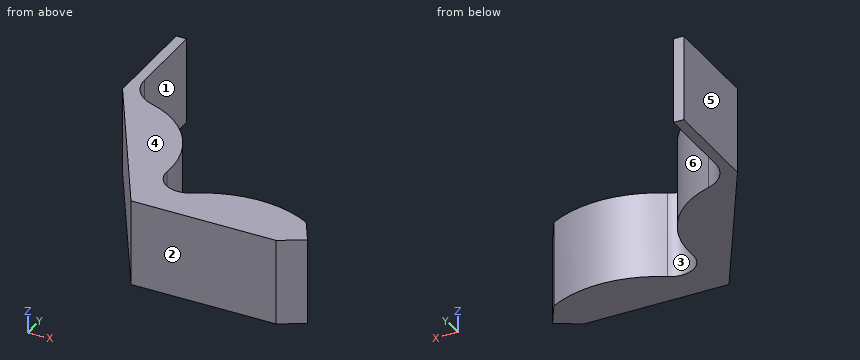
```python
from build123d import *

# Parameters (mm, degrees)
BOSS_EXTRUDE1_DEPTH = 250


with BuildPart() as part:
    # Sketch2 → Boss-Extrude1 (new body)
    with BuildSketch(Plane.XY):
        with BuildLine():
            Line((-277.128129211, 480), (0, 0))
            Line((0, 0), (420, 0))
            Line((420, 0), (489.282032303, 40))
            Line((489.282032303, 40), (445.980762114, 115))
            ThreePointArc((445.980762114, 115), (282.530694349, 155.502719239), (121.149011162, 107.415847331))
            ThreePointArc((121.149011162, 107.415847331), (48.13293846, 106.892445498), (14.374916134, 171.638231083))
            ThreePointArc((14.374916134, 171.638231083), (-32.686291511, 343.220804781), (-176.282688884, 448.270371763))
            ThreePointArc((-176.282688884, 448.270371763), (-227.488119154, 484.4090757), (-247.128129211, 543.926065009))
            Line((-247.128129211, 543.926065009), (-247.128129211, 775))
            Line((-247.128129211, 775), (-277.128129211, 775))
            Line((-277.128129211, 775), (-277.128129211, 480))
        make_face()
    extrude(amount=BOSS_EXTRUDE1_DEPTH)


solid = part.part
```
Source: CAD feature listing. Evaluate the final solid. Frame: model axes, mm. Face numbers are marked on the shaded views. A direction names the side the tool comes from. Coordinates: 2 decimals unless noted, no trailing zeros. Write each loop counter-clockwise with the first axis right and the second up, starting at its lowest first coordinate (ties: lowest second). Pieces come first, ordered by that corner, then holes. Notation, with made-up numbers: (-18.75, -38) -> (14.25, -38) arc R20 cw to (14.25, -13) -> close; hole circle Ø11 at (7, -12.75). An arc over 180 degrees is marked (long way). Return JSON: item names as keys, results as strings. Group by question number.
1) Section query A-A, the plane z = 121. Return loops of the section in (x, y), plus the area to 3 significant figures.
2) Ray query, line 1 along X through (y, z) = (583.5, 91); line 2 along Y through (x, z) = (89.5, 203.5); line 3 along X through (y, z) = (480, 120). Return the intervals inside material, ascending.
3) Section query B-B, the plane y = 564. Return loops of the section in (x, z).
4) Section query C-C, the plane x = 60. Return loops of the section in (y, z), plus the area to 3 significant figures.
5) Contact query for flat-ended pins moving along their axis: P1, Ø1.5, axis at x = 182.5, z = 128.5, coming from the +Y side; P2, Ø8, axis at y = 80.5, z = 190, coming from the +X side; P3, Ø2, axis at x = 203.5, z = 202.5, coming from the +Y side. Output: stop coordinate, or through.
6) Mould query, pull axis X, two halves, no side actions, for the marked faces 3, 4, 5 and 6. Classes: +X half, -X half, draft (parallel to the pull), parting line (faces both ways), or undercut.
7) Set-up query: the marked faces 1 and 2. Return all of +Z, -Z, +X, -X, +Y, -Y with unobstructed straight access to the full face (end or side cutting, diameter ignored); none if empty.
From the geometry:
{
 "1": {"outline": "(-277.13, 480) -> (0, 0) -> (420, 0) -> (489.28, 40) -> (445.98, 115) arc R320 ccw to (121.15, 107.42) arc R70 cw to (14.37, 171.64) arc R270 ccw to (-176.28, 448.27) arc R100 cw to (-247.13, 543.93) -> (-247.13, 775) -> (-277.13, 775) -> close", "area": "122,000 mm²"},
 "2": {"line 1": "-277.13 to -247.13", "line 2": "0 to 97.08", "line 3": "-277.13 to -224.03"},
 "3": {"outline": "(-277.13, 0) -> (-247.13, 0) -> (-247.13, 250) -> (-277.13, 250) -> close"},
 "4": {"outline": "(0, 0) -> (101.2, 0) -> (101.2, 250) -> (0, 250) -> close", "area": "25,300 mm²"},
 "5": {"P1": "y = 137.26", "P2": "x = 468.21", "P3": "y = 143.96"},
 "6": {"face 3": "undercut", "face 4": "draft", "face 5": "-X half", "face 6": "+X half"},
 "7": {"face 1": "+Z, -Z, +X, +Y", "face 2": "+Z, -Z, +X, -X, -Y"}
}
